```python
from build123d import *

# Parameters (mm, degrees)
F0_W     = 38.1
F0_H     = 38.1
F1_DEPTH = 1.27
F2_R     = 1.27
F3_DEPTH = 25.4
F4_R     = 1.5875
F5_DEPTH = 25.4


with BuildPart() as f1:
    # F0 (on Top) → F1 (new body)
    with BuildSketch(Plane.XY):
        Rectangle(F0_W, F0_H)
    extrude(amount=F1_DEPTH)

    # F2 (on Top) → F3 (cut)
    with BuildSketch(Plane.XY):
        Circle(F2_R)
    extrude(amount=F3_DEPTH, mode=Mode.SUBTRACT)

    # F4 (on Top) → F5 (cut)
    with BuildSketch(Plane.XY):
        with Locations((13.97, 13.97)):
            Circle(F4_R)
    extrude(amount=F5_DEPTH, mode=Mode.SUBTRACT)

    # F6: F1 across plane


with BuildPart() as f1_1:
    add(f1.part)
    add(f1.part.mirror(Plane.YZ), mode=Mode.INTERSECT)

    # F7: F1 across plane


with BuildPart() as f1_2:
    add(f1_1.part)
    add(f1_1.part.mirror(Plane.XZ), mode=Mode.INTERSECT)


solid = f1_2.part
```
Verification items for the finished model (mm, model axes). Round coordinates to 2 decimals unless told otherwise and drop trailing zeros. Loops run counter-clockwise (first coordinate to the right, second up) from the corner with the lowest first, then second, coordinate; pieces in that order, holes last. Notation, with made-up numbers: (73, 23.5) -> (109, 23.5) arc R21 cw to (109, 27.5) -> close; hole circle Ø6 at (76.25, -5.5). An arc over 180 degrees is marked (long way). Answer as a JSON object with one key per item and string values.
Q1. Section check B-B (z = 0.45). State how many separate pieces and enclosed holes the cut face has, then the cut area to 3 significant figures.
Data:
{"separate pieces": "1", "enclosed holes": "5", "area": "1,410 mm2"}
Q2. Draft check along Y on faces 1 (the cylindrical face through (15.436, -13.362, 0.626)), 2 (the flat face through (-19.05, 0, 1)), 3 (the flat face through (0, -19.05, 1)). Enter one of: pulls with the +Y half, pulls with the -Y half, needs draft (parallel to the pull), parting line crosses it, or undercut.
Data:
{"face 1": "undercut", "face 2": "needs draft", "face 3": "pulls with the -Y half"}
Q3. Section check A-A (y = 13.97). Record the boundary of the cut face in (x, z).
Data:
{"outline": "(-19.05, 0) -> (-15.56, 0) -> (-15.56, 1.27) -> (-19.05, 1.27) -> close; (-12.38, 0) -> (12.38, 0) -> (12.38, 1.27) -> (-12.38, 1.27) -> close; (15.56, 0) -> (19.05, 0) -> (19.05, 1.27) -> (15.56, 1.27) -> close"}
Q4. Scan lines: line 1 (X direction, y = 13.97, z = 0.75); line 2 (X direction, y = 0, z = 0.45). Record each from-to range of solid material in increasing order. Write a range as from..to.
Data:
{"line 1": "x = -19.05..-15.56, -12.38..12.38, 15.56..19.05", "line 2": "x = -19.05..-1.27, 1.27..19.05"}
Q5. Section check C-C (y = 0). Record the boundary of the cut face in (x, z), then the cut area to 3 significant figures.
Data:
{"outline": "(-19.05, 0) -> (-1.27, 0) -> (-1.27, 1.27) -> (-19.05, 1.27) -> close; (1.27, 0) -> (19.05, 0) -> (19.05, 1.27) -> (1.27, 1.27) -> close", "area": "45.2 mm2"}
